The figure shows three views and two pictorial views of one solid part (mm, origin at its lowest corner). Answer the questions. A direction names the side the tool comes from. Coordinates: 2 decimals unless noted, no trailing zeros. Write each loop counter-clockwise with the first axis right and the second up, starting at its lowest first coordinate (ties: lowest second). Pieces come first, ordered by that corner, then holes.
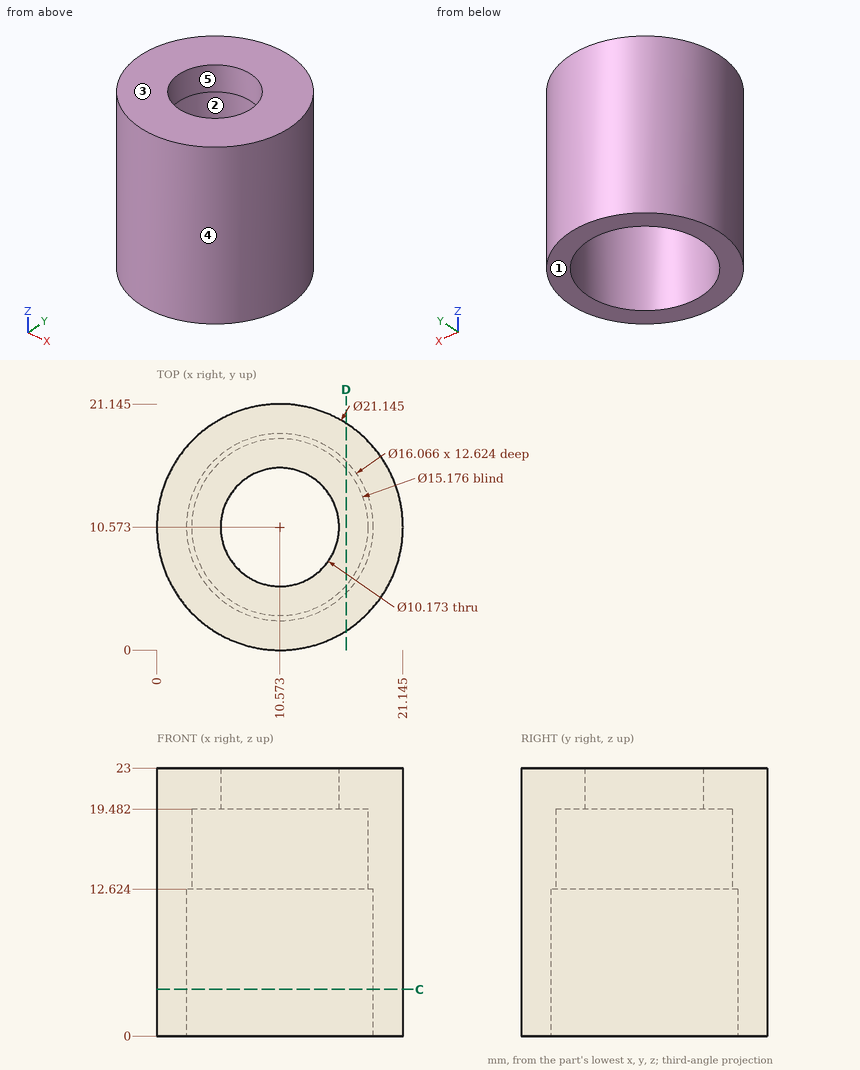
1. For a pull along Y with two mould halves and no side action, classify the marked faces 3, 4 and 5 as pulls with the +Y half, pulls with the -Y half, needs draft (parallel to the pull), parting line crosses it, or undercut.
Results found:
face 3: needs draft
face 4: parting line crosses it
face 5: undercut
2. Section C-C on z = 4 is taken. Give the vertices of the cut face in (x, y) (1 decimal).
Results found:
outline: circle Ø21.1 at (10.6, 10.6); hole circle Ø16.1 at (10.6, 10.6)
3. Find the intervals of material crossed by L1, parallel to Y at x = 10.75, z = 15; L2, parallel to Z at x = 17, y = 15.25; L3, parallel to Y at x = 12, z = 9.5, in increasing order.
Results found:
L1: y = 0 to 2.99, 18.16 to 21.14
L2: z = 12.62 to 23
L3: y = 0.1 to 2.67, 18.48 to 21.05
4. Section D-D on x = 16.25 is taken. Give the vertices of the cut face in (y, z) (1 decimal), then the cut area to 3 significant figures.
Results found:
outline: (1.7, 0) - (4.9, 0) - (4.9, 12.6) - (5.5, 12.6) - (5.5, 19.5) - (15.6, 19.5) - (15.6, 12.6) - (16.3, 12.6) - (16.3, 0) - (19.5, 0) - (19.5, 23) - (1.7, 23) - close
area: 198 mm2
5. A tool of negligible diameter and unlimited length cuts with its end or side. For the marked faces 1 and 2, from which of +Z, -Z, +X, -X, +Y, -Y can it reach the whole face along a straight path? Write none if from no direction.
Results found:
face 1: -Z, +X, -X, +Y, -Y
face 2: -Z
6. Flat-ended cylindrical pins translate along their axes: P1, Ø2, axis at y = 14.5, z = 14.5, coming from the -X side; P2, Ø1.5, axis at y = 14.5, z = 17.5, coming from the +X side; P3, Ø1, axis at y = 2.5, z = 17.5, coming from the -X side (1 decimal). Find the tip coordinate at first contact, or state that the pin passes through.
Results found:
P1: stops at x = 0.41
P2: stops at x = 20.66
P3: stops at x = 3.2
